```python
from build123d import *

# Parameters (mm, degrees)
SKETCH1_R           = 56.486183981
SKETCH1_R_2         = 22.440533472
BOSS_EXTRUDE1_DEPTH = 10
CUT_EXTRUDE1_DEPTH  = 2
CIRPATTERN1_COUNT   = 8


with BuildPart() as part:
    # Sketch1 → Boss-Extrude1 (new body)
    with BuildSketch(Plane(origin=(0, 0, 0), x_dir=(1, 0, 0), z_dir=(0, 1, 0))):
        Circle(SKETCH1_R)
        Circle(SKETCH1_R_2, mode=Mode.SUBTRACT)
    extrude(amount=BOSS_EXTRUDE1_DEPTH)

    # Sketch2 → Cut-Extrude1 (cut)
    with BuildSketch(Plane(origin=(0, 10, 0), x_dir=(1, 0, 0), z_dir=(0, 1, 0))):
        with BuildLine():
            Line((-9.135137375, 55.742607096), (-1.420081042, 3.855253414))
            ThreePointArc((-1.420081042, 3.855253414), (-0.302945279, 4.097295841), (0.837640155, 4.022184484))
            Line((0.837640155, 4.022184484), (0.837640155, 56.479972908))
            ThreePointArc((0.837640155, 56.479972908), (-4.165098092, 56.332414635), (-9.135137375, 55.742607096))
        make_face()
    cut_extrude1 = extrude(amount=-CUT_EXTRUDE1_DEPTH, mode=Mode.SUBTRACT)

    # CirPattern1: Cut-Extrude1 ×8 about axis
    cirpattern1_axis = Axis((0, 0, 0), (0, 1, 0))
    for i in range(1, CIRPATTERN1_COUNT):
        add(cut_extrude1.rotate(cirpattern1_axis, i * 360 / CIRPATTERN1_COUNT), mode=Mode.SUBTRACT)


solid = part.part
```
Model file for the job. Use its own axes, mm. A direction names the side the tool comes from. Give positions to 0.01 mm unless a question says otherwise; leave off trailing zeros. Order: outer loops, then holes, each group sorted by start corner. A loop starts at its lowest first (then second) coordinate and runs counter-clockwise, first axis right, second up.
1) Pin check, flat tips, straight feed: pin 1 (5 mm diameter, centred on x = 37.5, y = 5, fed in from +Z); pin 2 (2 mm diameter, centred on y = 9, z = -45.5, fed in from -X); pin 3 (2 mm diameter, centred on x = -18.5, y = 3, fed in from +Z). Stop position of each tip, or through.
2) 3-axis set-ups, long thin cutter, end or side, ignore diameter. For faces 1 (the flat face through (-1, 0, 24)), 2 (the flat face through (3, 8, 40)), 3 (the flat face through (-39.136, 9.014, 6.666)), 4 (the flat face through (27.136, 9.014, 28.321)): which of +Z, -Z, +X, -X, +Y, -Y reach the whole face in a straight line?
3) Mould opens along Z. For faces 5 (the flat face through (40, 8, -3)), 6 (the flat face through (-6.666, 9.014, -39.136)), 7 (the flat face through (36, 10, -18)) say: +Z half, -Z half, draft (parallel to the pull), parting line (faces both ways), or undercut.
4) Wall check: probe 1 along X at (y, z) = (7.25, 0); probe 2 along X at (y, z) = (8.75, -17). Give the ranges that are in metal, low to high.
5) Saw through at A-A, the plane z = 35.5. Write the cut outline in (x, y), then the cut area to 3 significant figures.
6) Saw through at C-C, the plane z = -38. Write the cut outline in (x, y), then the cut area to 3 significant figures.
7) Saw through at B-B, the plane y = 3.25. Write the cut outline in (x, z).
Computed:
1. pin 1: stops at z = 44.34
1. pin 2: stops at x = -34.79
1. pin 3: stops at z = 53.71
2. face 1: +Z, -Z, +X, -X, -Y
2. face 2: +Z, +Y
2. face 3: -X, +Y
2. face 4: +Y
3. face 5: undercut
3. face 6: -Z half
3. face 7: draft
4. probe 1: x = -56.49 to -22.44, 22.44 to 56.49
4. probe 2: x = -53.87 to -24.35, -15.82 to -14.65, 18.18 to 53.87
5. outline: (-43.94, 0) - (43.94, 0) - (43.94, 8) - (34.32, 8) - (34.32, 10) - (6.13, 10) - (6.13, 8) - (-0.84, 8) - (-0.84, 10) - (-25.27, 10) - (-25.27, 8) - (-36.68, 8) - (-36.68, 10) - (-43.94, 10) - close
5. area: 823 mm2
6. outline: (-41.79, 0) - (41.79, 0) - (41.79, 10) - (39.18, 10) - (39.18, 8) - (27.12, 8) - (27.12, 10) - (0.84, 10) - (0.84, 8) - (-6.5, 8) - (-6.5, 10) - (-36.82, 10) - (-36.82, 8) - (-41.79, 8) - close
6. area: 787 mm2
7. outline: circle Ø112.97 at (0, 0); hole circle Ø44.88 at (0, 0)
